from build123d import *

# Parameters (mm, degrees)
SKETCH_9_W                                     = 111
SKETCH_9_H                                     = 84
BOTTOM_BASE_1P5MM_FULL_111X84_DEPTH            = 1.5
SKETCH_10_W                                    = 101
SKETCH_10_H                                    = 74
SKETCH_10_R                                    = 3
BOTTOM_CENTER_FULL_THICKNESS_EXCEPT_STAN_DEPTH = 3
SKETCH_11_W                                    = 111
SKETCH_11_H                                    = 2
BOTTOM_OUTER_FRONT_OVERHANG_FULL_3MM_DEPTH     = 3
SKETCH_12_W                                    = 111
SKETCH_12_H                                    = 2
BOTTOM_OUTER_REAR_OVERHANG_FULL_3MM_DEPTH      = 3
SKETCH_13_W                                    = 2
SKETCH_13_H                                    = 80
BOTTOM_OUTER_LEFT_OVERHANG_FULL_3MM_DEPTH      = 3
SKETCH_14_W                                    = 2
SKETCH_14_H                                    = 80
BOTTOM_OUTER_RIGHT_OVERHANG_FULL_3MM_DEPTH     = 3
SKETCH_16_R                                    = 1.5
BOTTOM_M3_THROUGH_3MM_DEPTH                    = 1.5
SKETCH_18_R                                    = 16.5
BOTTOM_BATTERY_THROUGH_CLEARANCE_DEPTH         = 3
SKETCH_20_W                                    = 23
SKETCH_20_H                                    = 23
BOTTOM_BUZZER_THROUGH_CUT_DEPTH                = 3
SKETCH_21_R                                    = 1.5
BOTTOM_CENTER_RAIL_M3_THROUGH_3MM_DEPTH        = 6
BOTTOM_FILL_OLD_REAR_RABBET_1P5MM_START        = 1.5
SKETCH_22_W                                    = 101
SKETCH_22_H                                    = 1.5
BOTTOM_FILL_OLD_REAR_RABBET_1P5MM_DEPTH        = 1.5
SKETCH_23_W                                    = 107
SKETCH_23_H                                    = 2
BOTTOM_NEW_REAR_RABBET_1P5MM_DEEP_DEPTH        = 1.5
SKETCH_24_W                                    = 111
SKETCH_24_H                                    = 1.5
BOTTOM_REAR_OVERHANG_EXTENSION_1P5MM_DEPTH     = 3
TOOL_D3_R1P5_BUZZER_CORNERS_R                  = 1.5
BOTTOM_REAR_RABBET_WIDTH_FIX_3MM_START         = 1.5
SKETCH_25_W                                    = 107
SKETCH_25_H                                    = 0.5
BOTTOM_REAR_RABBET_WIDTH_FIX_3MM_DEPTH         = 1.5
TOOL_D3_R1P5_BOTTOM_RABBET_OUTER_CORNERS_R     = 1.5


with BuildPart() as part:
    # Sketch 9 → bottom_base_1p5mm_full_111x84 (new body)
    with BuildSketch(Plane.XY):
        with Locations((53.5, 40)):
            Rectangle(SKETCH_9_W, SKETCH_9_H)
    extrude(amount=BOTTOM_BASE_1P5MM_FULL_111X84_DEPTH)

    # Sketch 10 → bottom_center_full_thickness_except_stan (add)
    with BuildSketch(Plane.XY):
        with Locations((53.5, 40)):
            Rectangle(SKETCH_10_W, SKETCH_10_H)
        with Locations(Location((11.04, 7.54, 0), (0, 0, 180))):
            Circle(SKETCH_10_R, mode=Mode.SUBTRACT)
        with Locations(Location((95.96, 7.54, 0), (0, 0, 180))):
            Circle(SKETCH_10_R, mode=Mode.SUBTRACT)
        with Locations(Location((11.04, 72.46, 0), (0, 0, 180))):
            Circle(SKETCH_10_R, mode=Mode.SUBTRACT)
        with Locations(Location((95.96, 72.46, 0), (0, 0, 180))):
            Circle(SKETCH_10_R, mode=Mode.SUBTRACT)
    extrude(amount=BOTTOM_CENTER_FULL_THICKNESS_EXCEPT_STAN_DEPTH)

    # Sketch 11 → bottom_outer_front_overhang_full_3mm (add)
    with BuildSketch(Plane.XY):
        with Locations((53.5, -1)):
            Rectangle(SKETCH_11_W, SKETCH_11_H)
    extrude(amount=BOTTOM_OUTER_FRONT_OVERHANG_FULL_3MM_DEPTH)

    # Sketch 12 → bottom_outer_rear_overhang_full_3mm (add)
    with BuildSketch(Plane.XY):
        with Locations((53.5, 81)):
            Rectangle(SKETCH_12_W, SKETCH_12_H)
    extrude(amount=BOTTOM_OUTER_REAR_OVERHANG_FULL_3MM_DEPTH)

    # Sketch 13 → bottom_outer_left_overhang_full_3mm (add)
    with BuildSketch(Plane.XY):
        with Locations((-1, 40)):
            Rectangle(SKETCH_13_W, SKETCH_13_H)
    extrude(amount=BOTTOM_OUTER_LEFT_OVERHANG_FULL_3MM_DEPTH)

    # Sketch 14 → bottom_outer_right_overhang_full_3mm (add)
    with BuildSketch(Plane.XY):
        with Locations((108, 40)):
            Rectangle(SKETCH_14_W, SKETCH_14_H)
    extrude(amount=BOTTOM_OUTER_RIGHT_OVERHANG_FULL_3MM_DEPTH)

    # Sketch 16 → bottom_m3_through_3mm (cut)
    with BuildSketch(Plane.XY):
        with Locations(Location((11.04, 7.54, 0), (0, 0, 180))):
            Circle(SKETCH_16_R)
        with Locations(Location((95.96, 7.54, 0), (0, 0, 180))):
            Circle(SKETCH_16_R)
        with Locations(Location((11.04, 72.46, 0), (0, 0, 180))):
            Circle(SKETCH_16_R)
        with Locations(Location((95.96, 72.46, 0), (0, 0, 180))):
            Circle(SKETCH_16_R)
    extrude(amount=BOTTOM_M3_THROUGH_3MM_DEPTH, mode=Mode.SUBTRACT)

    # Sketch 18 → bottom_battery_through_clearance (cut)
    with BuildSketch(Plane.XY):
        with Locations(Location((58.8, 24.5, 0), (0, 0, 180))):
            Circle(SKETCH_18_R)
    extrude(amount=BOTTOM_BATTERY_THROUGH_CLEARANCE_DEPTH, mode=Mode.SUBTRACT)

    # Sketch 20 → bottom_buzzer_through_cut (cut)
    with BuildSketch(Plane.XY):
        with Locations((32.4, 17.3)):
            Rectangle(SKETCH_20_W, SKETCH_20_H)
    extrude(amount=BOTTOM_BUZZER_THROUGH_CUT_DEPTH, mode=Mode.SUBTRACT)

    # Sketch 21 → bottom_center_rail_m3_through_3mm (cut)
    with BuildSketch(Plane.XY):
        with Locations(Location((8, 25, 0), (0, 0, 180))):
            Circle(SKETCH_21_R)
        with Locations(Location((8, 55, 0), (0, 0, 180))):
            Circle(SKETCH_21_R)
        with Locations(Location((99, 25, 0), (0, 0, 180))):
            Circle(SKETCH_21_R)
        with Locations(Location((99, 55, 0), (0, 0, 180))):
            Circle(SKETCH_21_R)
    extrude(amount=BOTTOM_CENTER_RAIL_M3_THROUGH_3MM_DEPTH, mode=Mode.SUBTRACT)

    # Sketch 22 → bottom_fill_old_rear_rabbet_1p5mm (add)
    with BuildSketch(Plane.XY.offset(BOTTOM_FILL_OLD_REAR_RABBET_1P5MM_START)):
        with Locations((53.5, 77.75)):
            Rectangle(SKETCH_22_W, SKETCH_22_H)
    extrude(amount=BOTTOM_FILL_OLD_REAR_RABBET_1P5MM_DEPTH)

    # Sketch 23 → bottom_new_rear_rabbet_1p5mm_deep (cut)
    with BuildSketch(Plane.XY.offset(3)):
        with Locations((53.5, 81)):
            Rectangle(SKETCH_23_W, SKETCH_23_H)
    extrude(amount=-BOTTOM_NEW_REAR_RABBET_1P5MM_DEEP_DEPTH, mode=Mode.SUBTRACT)

    # Sketch 24 → bottom_rear_overhang_extension_1p5mm (add)
    with BuildSketch(Plane.XY):
        with Locations((53.5, 82.75)):
            Rectangle(SKETCH_24_W, SKETCH_24_H)
    extrude(amount=BOTTOM_REAR_OVERHANG_EXTENSION_1P5MM_DEPTH)

    # tool_D3_R1p5_buzzer_corners
    tool_d3_r1p5_buzzer_corners_edges = [part.edges().sort_by_distance(p)[0] for p in [
        (42.870153799, 28.8, 1.5),
        (43.9, 17.411981941, 1.5),
        (20.9, 28.8, 1.5),
        (20.9, 5.8, 1.5),
        (43.9, 5.8, 1.5),
    ]]
    fillet(tool_d3_r1p5_buzzer_corners_edges, radius=TOOL_D3_R1P5_BUZZER_CORNERS_R)

    # Sketch 25 → bottom_rear_rabbet_width_fix_3mm (add)
    with BuildSketch(Plane.XY.offset(BOTTOM_REAR_RABBET_WIDTH_FIX_3MM_START)):
        with Locations((53.5, 81.75)):
            Rectangle(SKETCH_25_W, SKETCH_25_H)
    extrude(amount=BOTTOM_REAR_RABBET_WIDTH_FIX_3MM_DEPTH)

    # tool_D3_R1p5_bottom_rabbet_outer_corners
    tool_d3_r1p5_bottom_rabbet_outer_corners_edges = [part.edges().sort_by_distance(p)[0] for p in [
        (107, 0, 2.25),
        (0, 81.5, 2.25),
        (107, 81.5, 2.25),
        (0, 0, 2.25),
    ]]
    fillet(tool_d3_r1p5_bottom_rabbet_outer_corners_edges, radius=TOOL_D3_R1P5_BOTTOM_RABBET_OUTER_CORNERS_R)


solid = part.part
Could you check a few things on this model? Use its own coordinates, in mm. A direction names the side the tool comes from. Give positions to 0.01 mm unless a question says otherwise; leave off trailing zeros. Write each loop counter-clockwise with the first axis right and the second up, starting at its lowest first coordinate (ties: lowest second). Pieces come first, ordered by that corner, then holes. Notation, with made-up numbers: (87.5, 79.25) -> (143.5, 79.25) arc R27 ccw to (143.5, 96.25) -> close; hole circle Ø7 at (2, 72.25). An arc over 180 degrees is marked (long way). Answer as CSV lines item,"result". Start each with the question number.
(1) If we mould it in two halves opening along Y, with no side actions, what happens to faces 1 (the face through (53, 83.5, 1)), 2 (the face through (44.84, 13.873, 1.479)), 3 (the face through (-2, 40, 1))? For each: +Y half, -Y half, draft (parallel to the pull), parting line (faces both ways), or undercut.
(2) Please list where these lines run through material, in increasing order: line 1 (X direction, y = 72.46, z = 0.8); line 2 (X direction, y = 4.5, z = 2.9); line 3 (Y direction, x = 99, z = 2.3).
(3) If we section it at B-B, the plane x = 58.8: Write out the boundary of the cut face in (y, z).
(4) Which directions (+Z, -Z, +X, -X, +Y, -Y) give clear straight access to the entire face, cutting with the end or side of a thin tool? Please do faces 4 (the face through (53, -2, 1)), 5 (the face through (32, 5.8, 1)), 6 (the face through (11.431, 69.486, 2.24)).
(5) If we section it at C-C, the plane z = 2.45: Give the number of separate pieces and of enclosed holes in the cut face, and give its area (3 significant figures).
(6) If we section it at A-A, the plane y = 55: Write out the boundary of the cut face in (x, z), and give its area (3 significant figures).
(7) If we section it at D-D, the plane x = 95.96: Write out the boundary of the cut face in (y, z).
(8) I'm going to push flat-ended pins straight in: pin 1 Ø3.5 at (x, y) = (11.04, 7.54) entering from +Z; pin 2 Ø2.5 at (x, y) = (99, 25) entering from +Z. Where does each tip first touch, or does it pass through?
Answer list:
1,face 1,"+Y half"
1,face 2,"undercut"
1,face 3,"draft"
2,line 1,"-2 to 9.54, 12.54 to 94.46, 97.46 to 109"
2,line 2,"-2 to 0, 3 to 104, 107 to 109"
2,line 3,"-2 to 0, 3 to 23.5, 26.5 to 53.5, 56.5 to 78.5, 81.5 to 83.5"
3,outline,"(-2, 0) -> (8, 0) -> (8, 3) -> (3, 3) -> (3, 1.5) -> (0, 1.5) -> (0, 3) -> (-2, 3) -> close; (41, 0) -> (83.5, 0) -> (83.5, 3) -> (81.5, 3) -> (81.5, 1.5) -> (78.5, 1.5) -> (78.5, 3) -> (41, 3) -> close"
4,face 4,"+Z, -Z, +X, -X, -Y"
4,face 5,"+Z, -Z"
4,face 6,"+Z"
5,separate pieces,"2"
5,enclosed holes,"10"
5,area,"6,880 mm^2"
6,outline,"(-2, 0) -> (6.5, 0) -> (6.5, 3) -> (3, 3) -> (3, 1.5) -> (0, 1.5) -> (0, 3) -> (-2, 3) -> close; (9.5, 0) -> (97.5, 0) -> (97.5, 3) -> (9.5, 3) -> close; (100.5, 0) -> (109, 0) -> (109, 3) -> (107, 3) -> (107, 1.5) -> (104, 1.5) -> (104, 3) -> (100.5, 3) -> close"
6,area,"306 mm^2"
7,outline,"(-2, 0) -> (6.04, 0) -> (6.04, 1.5) -> (4.54, 1.5) -> (4.54, 3) -> (3, 3) -> (3, 1.5) -> (0, 1.5) -> (0, 3) -> (-2, 3) -> close; (9.04, 0) -> (70.96, 0) -> (70.96, 1.5) -> (69.46, 1.5) -> (69.46, 3) -> (10.54, 3) -> (10.54, 1.5) -> (9.04, 1.5) -> close; (73.96, 0) -> (83.5, 0) -> (83.5, 3) -> (81.5, 3) -> (81.5, 1.5) -> (78.5, 1.5) -> (78.5, 3) -> (75.46, 3) -> (75.46, 1.5) -> (73.96, 1.5) -> close"
8,pin 1,"z = 1.5"
8,pin 2,"through"
